Here's how the part is built. I have some questions about the finished solid (model axes, mm). A direction names the side the tool comes from. Round coordinates to 2 decimals unless told otherwise and drop trailing zeros. Write each loop counter-clockwise with the first axis right and the second up, starting at its lowest first coordinate (ties: lowest second). Pieces come first, ordered by that corner, then holes. Notation, with made-up numbers: (68.25, 44) - (101.25, 44) arc R22 cw to (101.25, 77) - close; hole circle Ø7 at (-39.75, -13). An arc over 180 degrees is marked (long way). One line per item, written item: value. Start each with the question number.
Item 1: Thinking about a two-plate mould opening in Y: for faces 3 (the face through (36.316, -11.437, 1.565)), 4 (the face through (0.661, -25.712, 1.61)), 5 (the face through (-1, 1, 0)), 6 (the face through (22.37, 6.67, 3.22)), which applies, released by +Y, released by -Y, zero draft, split by the parting line, or undercut?
Item 2: If I drill on line 1 (Y direction, x = 0, z = 3.9); line 2 (Y direction, x = 0, z = 0.75); line 3 (X direction, y = 7.62, z = 4.75) (3 decimals), over which ranges is the centre line in solid material (lowest first)?
Item 3: For P1, Ø1, axis at x = -9, z = 4, coming from the +Y side; P2, Ø1.5, axis at y = -10.5, z = 5, coming from the -X side; P3, Ø1, axis at y = 2.5, z = 5.5, coming from the -X side, each with a flat end and sliding along its axis, tell me the tip position at first contact or that it passes through.
Item 4: Imagine slicing it at C-C, the plane x = -11.5. Please give me the cut outline in (y, z) (3 decimals), then the cut area to 3 significant figures.
Item 5: Imagine slicing it at B-B, the plane y = 7.62. Please give me the cut outline in (x, z) (3 decimals).
Item 6: Imagine slicing it at D-D, the plane y = 27.5. Please give me the cut outline in (x, z) (3 decimals), then the cut area to 3 significant figures.
Item 7: For faces 1 (the face through (1.11, -29.11, 4.78)), 2 (the face through (1, -1, 6.35)), which set-ups out of +Z, -Z, +X, -X, +Y, -Y let a thin tool reach every point of the face, with its end or its side?
Autodesk Fusion 360 part; units mm, degrees
sketch "Sketch1" plane through (0, 0, 0) normal (0, 0, 1) x (1, 0, 0)
  circle A0 centre (0, 0) radius 38.0746
  dimension "d1" = 76.1492
extrude "Extrude1" add sketch "Sketch1" along normal blind 3.175
sketch "Sketch2" plane through (0, 0, 3.175) normal (0, 0, 1) x (-1, 0, 0)
  circle A0 centre (0, 0) radius 38.0746
  circle A1 centre (0, 0) radius 36.5125
  dimension "d4" = 73.025
extrude "Extrude2" add sketch "Sketch2" along normal blind 3.175 contours A1
sketch "Sketch3" plane through (0, 0, 6.35) normal (0, 0, 1) x (-1, 0, 0)
  circle A0 centre (0, 0) radius 36.5125
  circle A1 centre (25.4, -7.62) radius 3.175
  circle A2 centre (-25.4, -7.62) radius 3.175
  circle A3 centre (0, 20.6756) radius 5.08
  circle A4 centre (0, 0) radius 38.0746
  dimension "d7" = 50.8
  dimension "d8" = 25.4
  dimension "d9" = 7.62
  dimension "d10" = 6.35
  dimension "d11" = 6.35
  dimension "d12" = 10.16
  dimension "d13" = 20.6756
extrude "Extrude3" cut sketch "Sketch3" against normal blind 6.35 contours A1 | A2 | A3
sketch "Sketch4" plane through (0, 0, 6.35) normal (0, 0, 1) x (-1, 0, 0)
  circle A0 centre (-25.4, -7.62) radius 3.175
  circle A1 centre (0, 20.6756) radius 5.08
  circle A2 centre (25.4, -7.62) radius 3.175
  circle A3 centre (0, 0) radius 36.5125
  circle A4 centre (0, 20.6756) radius 8.509
  dimension "d16" = 17.018
extrude "Extrude4" cut sketch "Sketch4" against normal blind 3.175 contours A4
equation "d2 = ( 0.25 / 2 ) * 1 in"
equation "d5 = ( 0.25 / 2 ) * 1 in"
Values follow:
1. face 3: split by the parting line
1. face 4: undercut
1. face 5: zero draft
1. face 6: undercut
2. line 1: y = -36.51 to -29.18, -12.17 to 36.51
2. line 2: y = -38.07 to -25.76, -15.6 to 38.07
2. line 3: x = -35.709 to -28.575, -22.225 to 22.225, 28.575 to 35.709
3. P1: stops at y = 35.51
3. P2: stops at x = -35.19
3. P3: stops at x = -36.46
4. outline: (-36.296, 0) - (36.296, 0) - (36.296, 3.175) - (34.654, 3.175) - (34.654, 6.35) - (-34.654, 6.35) - (-34.654, 3.175) - (-36.296, 3.175) - close
4. area: 451 mm^2
5. outline: (-37.304, 0) - (-28.575, 0) - (-28.575, 6.35) - (-35.709, 6.35) - (-35.709, 3.175) - (-37.304, 3.175) - close; (-22.225, 0) - (22.225, 0) - (22.225, 6.35) - (-22.225, 6.35) - close; (28.575, 0) - (37.304, 0) - (37.304, 3.175) - (35.709, 3.175) - (35.709, 6.35) - (28.575, 6.35) - close
6. outline: (-26.333, 0) - (26.333, 0) - (26.333, 3.175) - (24.019, 3.175) - (24.019, 6.35) - (-24.019, 6.35) - (-24.019, 3.175) - (-26.333, 3.175) - close
6. area: 320 mm^2
7. face 1: +Z
7. face 2: +Z, +X, -X, +Y, -Y
